Check sheet for the modelled part. Datum: model origin and axes. Units: mm. Give positions to 0.01 mm unless a question says otherwise; leave off trailing zeros. Loops run counter-clockwise (first coordinate to the right, second up) from the corner with the lowest first, then second, coordinate; pieces in that order, holes last. Notation, with made-up numbers: (0, 64.5) - (17, 64.5) arc R22 ccw to (17, 103.5) - close; hole circle Ø2 at (-15, 45). An arc over 180 degrees is marked (long way). Use one line per item in the form item = value.
from build123d import *

# Parameters (mm, degrees)
SKETCH1_R               = 25
BOSS_EXTRUDE1_DEPTH     = 200
SKETCH2_R               = 30
BOSS_EXTRUDE2_DEPTH     = 30
FILLET1_R               = 10
FILLET2_R               = 2
CHAMFER1_SIZE           = 5
CUT_EXTRUDE1_DEPTH      = 234.880311271
CUT_EXTRUDE1_DEPTH_BACK = 234.880311271
SKETCH3_R               = 2.5


with BuildPart() as part:
    # Sketch1 → Boss-Extrude1 (new body)
    with BuildSketch(Plane.XY):
        Circle(SKETCH1_R)
    extrude(amount=BOSS_EXTRUDE1_DEPTH)

    # Sketch2 → Boss-Extrude2 (add)
    with BuildSketch(Plane.XY.offset(200)):
        Circle(SKETCH2_R)
    extrude(amount=BOSS_EXTRUDE2_DEPTH)

    # Fillet1
    fillet1_edges = [part.edges().sort_by_distance(p)[0] for p in [
        (-30, 0, 230),
    ]]
    fillet(fillet1_edges, radius=FILLET1_R)

    # Fillet2
    fillet2_edges = [part.edges().sort_by_distance(p)[0] for p in [
        (-25, 0, 200),
        (-30, 0, 200),
    ]]
    fillet(fillet2_edges, radius=FILLET2_R)

    # Chamfer1
    chamfer1_edges = [part.edges().sort_by_distance(p)[0] for p in [
        (-25, 0, 0),
    ]]
    chamfer(chamfer1_edges, length=CHAMFER1_SIZE)

    # Sketch3 → Cut-Extrude1 (cut, two sides: drawn at the far end of the back side and taken through both)
    with BuildSketch(Plane(origin=(0, 0, 0), x_dir=(1, 0, 0), z_dir=(0, 1, 0)).offset(-CUT_EXTRUDE1_DEPTH_BACK)):
        with Locations(Location((0, -45, 0), (0, 0, 270))):
            Circle(SKETCH3_R)
    extrude(amount=CUT_EXTRUDE1_DEPTH + CUT_EXTRUDE1_DEPTH_BACK, mode=Mode.SUBTRACT)


solid = part.part
Item 1: Section check C-C on z = 29. Record the boundary of the cut face in (x, y), then the cut area to 3 significant figures.
Answer block:
outline = circle Ø50 at (0, 0)
area = 1,960 mm2
Item 2: Mould release check, pull along X, two halves, no side actions. Record for faces 1 (the face through (-0.96, -0.35, 47.31)), 2 (the face through (-15, 23, 200)), 3 (the face through (23.846, 7.509, 100.149)): released by +X, released by -X, zero draft, split by the parting line, or undercut.
Answer block:
face_1 = undercut
face_2 = zero draft
face_3 = split by the parting line
Item 3: Section check A-A on x = 0. Record the boundary of the cut face in (y, z), then the cut area to 3 significant figures.
Answer block:
outline = (-30, 202) arc R2 ccw to (-28, 200) - (-27, 200) arc R2 cw to (-25, 198) - (-25, 47.5) - (25, 47.5) - (25, 198) arc R2 cw to (27, 200) - (28, 200) arc R2 ccw to (30, 202) - (30, 220) arc R10 ccw to (20, 230) - (-20, 230) arc R10 ccw to (-30, 220) - close; (-25, 5) - (-20, 0) - (20, 0) - (25, 5) - (25, 42.5) - (-25, 42.5) - close
area = 11,500 mm2
Item 4: Section check B-B on y = 0. Record the boundary of the cut face in (x, z), then the cut area to 3 significant figures.
Answer block:
outline = (-30, 202) arc R2 ccw to (-28, 200) - (-27, 200) arc R2 cw to (-25, 198) - (-25, 5) - (-20, 0) - (20, 0) - (25, 5) - (25, 198) arc R2 cw to (27, 200) - (28, 200) arc R2 ccw to (30, 202) - (30, 220) arc R10 ccw to (20, 230) - (-20, 230) arc R10 ccw to (-30, 220) - close; hole circle Ø5 at (0, 45)
area = 11,700 mm2
Item 5: Thickness scan on L1, parallel to Z at x = 0, y = 13; L2, parallel to X at y = 7.5, z = 45; L3, parallel to Z at x = -0.5, y = 21.5. Record the ranges inside material, lowest first.
Answer block:
L1 = 0 to 42.5, 47.5 to 230
L2 = -23.85 to -2.5, 2.5 to 23.85
L3 = 1.51 to 42.55, 47.45 to 229.89
Item 6: Gauge pin test, flat ends, axial feed: P1, Ø5, axis at x = 14.5, z = 175, coming from the +Y side; P2, Ø2, axis at x = -3, z = 146, coming from the -Y side; P3, Ø12, axis at x = 9, z = 190, coming from the -Y side; P4, Ø3, axis at x = 0, z = 45, coming from the +Y side. Record the tip position at first contact, or that the pin passes through.
Answer block:
P1 = 21.93
P2 = -24.92
P3 = -24.82
P4 = through
